```python
from build123d import *

# Parameters (mm, degrees)
SKETCH015_W             = 74.9
SKETCH015_H             = 3.5
PAD002_DEPTH            = 5
SKETCH017_W             = 5.35
SKETCH017_H             = 49
PAD003_DEPTH            = 10
LINEARPATTERN004_COUNT  = 11
LINEARPATTERN004_PITCH  = 6.955
CHAMFER_SIZE            = 0.6
BODY002_PLACEMENT_ANGLE = 90


with BuildPart() as part:
    # Sketch015 → Pad002 (new body)
    with BuildSketch(Plane.XY):
        with Locations((37.45, -1.75)):
            Rectangle(SKETCH015_W, SKETCH015_H)
    extrude(amount=-PAD002_DEPTH)

    # Sketch017 → Pad003 (join)
    with BuildSketch(Plane.XZ):
        with Locations((2.675, 24.5)):
            Rectangle(SKETCH017_W, SKETCH017_H)
    pad003 = extrude(amount=PAD003_DEPTH)

    # LinearPattern004: Pad003 ×11
    with Locations(*[(i * LINEARPATTERN004_PITCH, 0, 0) for i in range(1, LINEARPATTERN004_COUNT)]):
        add(pad003)

    # Chamfer
    chamfer_edges = [part.edges().sort_by_distance(p)[0] for p in [
        (2.675, -10, 0),
        (5.35, -10, 24.5),
        (2.675, -10, 49),
        (0, -10, 24.5),
        (9.63, -10, 0),
        (12.305, -10, 24.5),
        (9.63, -10, 49),
        (6.955, -10, 24.5),
        (16.585, -10, 0),
        (19.26, -10, 24.5),
        (16.585, -10, 49),
        (13.91, -10, 24.5),
        (23.54, -10, 0),
        (26.215, -10, 24.5),
        (23.54, -10, 49),
        (20.865, -10, 24.5),
        (30.495, -10, 0),
        (33.17, -10, 24.5),
        (30.495, -10, 49),
        (27.82, -10, 24.5),
        (37.45, -10, 0),
        (40.125, -10, 24.5),
        (37.45, -10, 49),
        (34.775, -10, 24.5),
        (44.405, -10, 0),
        (47.08, -10, 24.5),
        (44.405, -10, 49),
        (41.73, -10, 24.5),
        (51.36, -10, 0),
        (54.035, -10, 24.5),
        (51.36, -10, 49),
        (48.685, -10, 24.5),
        (58.315, -10, 0),
        (60.99, -10, 24.5),
        (58.315, -10, 49),
        (55.64, -10, 24.5),
        (65.27, -10, 0),
        (67.945, -10, 24.5),
        (65.27, -10, 49),
        (62.595, -10, 24.5),
        (72.225, -10, 0),
        (74.9, -10, 24.5),
        (72.225, -10, 49),
        (69.55, -10, 24.5),
        (0, 0, 22),
        (2.675, 0, 49),
        (5.35, 0, 24.5),
        (6.1525, 0, 0),
        (6.955, 0, 24.5),
        (9.63, 0, 49),
        (12.305, 0, 24.5),
        (13.1075, 0, 0),
        (13.91, 0, 24.5),
        (16.585, 0, 49),
        (19.26, 0, 24.5),
        (20.0625, 0, 0),
        (20.865, 0, 24.5),
        (23.54, 0, 49),
        (26.215, 0, 24.5),
        (27.0175, 0, 0),
        (27.82, 0, 24.5),
        (30.495, 0, 49),
        (33.17, 0, 24.5),
        (33.9725, 0, 0),
        (34.775, 0, 24.5),
        (37.45, 0, 49),
        (40.125, 0, 24.5),
        (40.9275, 0, 0),
        (41.73, 0, 24.5),
        (44.405, 0, 49),
        (47.08, 0, 24.5),
        (47.8825, 0, 0),
        (48.685, 0, 24.5),
        (51.36, 0, 49),
        (54.035, 0, 24.5),
        (54.8375, 0, 0),
        (55.64, 0, 24.5),
        (58.315, 0, 49),
        (60.99, 0, 24.5),
        (61.7925, 0, 0),
        (62.595, 0, 24.5),
        (65.27, 0, 49),
        (67.945, 0, 24.5),
        (68.7475, 0, 0),
        (69.55, 0, 24.5),
        (72.225, 0, 49),
        (74.9, 0, 22),
        (37.45, 0, -5),
        (5.35, -5, 49),
        (0, -5, 49),
        (12.305, -5, 49),
        (6.955, -5, 49),
        (19.26, -5, 49),
        (13.91, -5, 49),
        (26.215, -5, 49),
        (20.865, -5, 49),
        (33.17, -5, 49),
        (27.82, -5, 49),
        (40.125, -5, 49),
        (34.775, -5, 49),
        (47.08, -5, 49),
        (41.73, -5, 49),
        (54.035, -5, 49),
        (48.685, -5, 49),
        (60.99, -5, 49),
        (55.64, -5, 49),
        (67.945, -5, 49),
        (62.595, -5, 49),
        (74.9, -5, 49),
        (69.55, -5, 49),
        (74.9, -1.75, -5),
        (37.45, -3.5, -5),
        (0, -1.75, -5),
    ]]
    chamfer(chamfer_edges, length=CHAMFER_SIZE)


with BuildPart() as part_1:
    # Body002 placement: moved
    add(part.part.rotate(Axis((0, 0, 0), (-1, 0, 0)), BODY002_PLACEMENT_ANGLE))


solid = part_1.part
```
Input: part model. Units: mm. Frame: model coordinates. A direction names the side the tool comes from. Give positions to 0.01 mm unless a question says otherwise; leave off trailing zeros. Write each loop counter-clockwise with the first axis right and the second up, starting at its lowest first coordinate (ties: lowest second). Pieces come first, ordered by that corner, then holes. Notation, with made-up numbers: (-36, 65) - (12, 65) arc R19 ccw to (12, 77) - close; hole circle Ø3 at (11, -34). An arc over 180 degrees is marked (long way). Write item = value, one per line. Start each with the question number.
1. Access query for faces 4 (the flat face through (37, -2, 3.5)), 5 (the flat face through (19.26, 24, 5)), 6 (the flat face through (37, -5, 2)). Directions: +Z, -Z, +X, -X, +Y, -Y. A direction counts if a zero-diameter tool reaches every point of the face in a straight line with its end or side. Return the directions, or none.
2. First-contact query: pin 1 Ø1.6 at (x, z) = (10.5, 5.5) entering from -Y; pin 2 Ø0.5 at (x, z) = (47.5, 2.5) entering from +Y; pin 3 Ø1.5 at (x, z) = (40.5, 4) entering from -Y. Flat tips, straight axial feed; report the tip coordinate or a pass-through.
3. Mould query, pull axis X, two halves, no side actions, for faces 1 (the flat face through (0, 22, 5)), 2 (the flat face through (30, 0, 6)), 3 (the flat face through (20, 0, 2)). Classes: released by +X, released by -X, zero draft, split by the parting line, or undercut.
4. Section query B-B, the plane y = 27.5. Count the separate pieces of the cut face and the enclosed holes in it, then the cut area to 3 significant figures.
5. Ray query, L1, parallel to Z at x = 63, y = -3; L2, parallel to Y at x = 19.5, z = 0.75; L3, parallel to Y at x = 22.5, z = 7.75. Return the intervals inside material, ascending.
6. Section query A-A, the plane x = 30. Output: boundary loops of the cut face in (y, z).
Check sheet entries:
q1.face_4 = +Z, +X, -X, -Y
q1.face_5 = +Z, -Z, +Y
q1.face_6 = +Z, -Z, +X, -X, -Y
q2.pin_1 = 0
q2.pin_2 = 0
q2.pin_3 = -4.65
q3.face_1 = released by -X
q3.face_2 = zero draft
q3.face_3 = undercut
q4.separate_pieces = 11
q4.enclosed_holes = 0
q4.area = 581 mm2
q5.L1 = 0 to 3.5
q5.L2 = -5 to 0
q5.L3 = 0 to 49
q6.outline = (-5, 0.6) - (-4.4, 0) - (48.4, 0) - (49, 0.6) - (49, 9.4) - (48.4, 10) - (0.6, 10) - (0, 9.4) - (0, 3.5) - (-4.4, 3.5) - (-5, 2.9) - close
